```python
from build123d import *

# Parameters (mm, degrees)
BOSS_EXTRUDE2_START = -109.568605
BOSS_EXTRUDE2_DEPTH = 101.325087
CIRPATTERN1_COUNT   = 8


with BuildPart() as part:
    # Sketch3 → Revolve1 (revolve)
    with BuildSketch(Plane(origin=(0, 0, 0), x_dir=(0, 0, -1), z_dir=(1, 0, 0))):
        Polygon((0, 120), (0, 0), (10, 0), (10, 4.243518426), (8, 4.243518426), (8, 8.243518426), (10, 8.243518426), (10, 109.568605079), (8, 109.568605079), (8, 113.568605079), (10, 113.568605079), (10, 120), align=None)
    revolve(axis=Axis((0, 0, 0), (0, 1, 0)))

    # Sketch4 → Boss-Extrude2 (add)
    with BuildSketch(Plane.XZ.offset(BOSS_EXTRUDE2_START)):
        with BuildLine():
            Line((-1, 9.949874371), (-1, 10.949874371))
            Line((-1, 10.949874371), (1, 10.949874371))
            Line((1, 10.949874371), (1, 9.949874371))
            ThreePointArc((1, 9.949874371), (0, 10), (-1, 9.949874371))
        make_face()
    boss_extrude2 = extrude(amount=BOSS_EXTRUDE2_DEPTH)

    # CirPattern1: Boss-Extrude2 ×8 about axis
    cirpattern1_axis = Axis((0, 0, 0), (0, 1, 0))
    for i in range(1, CIRPATTERN1_COUNT):
        add(boss_extrude2.rotate(cirpattern1_axis, i * 360 / CIRPATTERN1_COUNT))


solid = part.part
```
Could you check a few things on this model? Use its own coordinates, in mm. A direction names the side the tool comes from. Round coordinates to 2 decimals unless told otherwise and drop trailing zeros. Loops run counter-clockwise (first coordinate to the right, second up) from the corner with the lowest first, then second, coordinate; pieces in that order, holes last. Notation, with made-up numbers: (55, 28.5) - (80, 28.5) arc R19 cw to (80, 36.5) - close; hole circle Ø4 at (-11.75, 81.25). An arc over 180 degrees is marked (long way). Answer as CSV lines item,"result".
1. I want a section at A-A on z = 0. List the corners of the cut face in (x, y) for me.
Filled in:
outline,"(-10.95, 8.24) - (-8, 8.24) - (-8, 4.24) - (-10, 4.24) - (-10, 0) - (10, 0) - (10, 4.24) - (8, 4.24) - (8, 8.24) - (10.95, 8.24) - (10.95, 109.57) - (8, 109.57) - (8, 113.57) - (10, 113.57) - (10, 120) - (-10, 120) - (-10, 113.57) - (-8, 113.57) - (-8, 109.57) - (-10.95, 109.57) - close"
2. Please list where these lines run through material, in increasing order: line 1 along Y through (x, z) = (1.25, -9); line 2 along X through (y, z) = (43, 8.25); line 3 along Z through (x, y) = (-8, 77.5). Write a range as [from, to].
Filled in:
line 1,"y = [0, 4.24], [8.24, 109.57], [113.57, 120]"
line 2,"x = [-7.24, -6.84], [-5.65, 5.65], [6.84, 7.24]"
line 3,"z = [-7.49, -6.59], [-6, 6], [6.59, 7.49]"
3. We'd pull the mould along Y, two halves only. Please class faces 6 (the face through (0, 0, 0)), 7 (the face through (3.789, 59.615, 9.254)), 8 (the face through (-8.2, 113.569, 0)): +Y half, -Y half, draft (parallel to the pull), parting line (faces both ways), or undercut.
Filled in:
face 6,"-Y half"
face 7,"draft"
face 8,"undercut"
4. On a 3-axis mill with a long thin cutter (end or side, diameter ignored), from which of +Z, -Z, +X, -X, +Y, -Y can I reach the whole of each face in a straight line? I mean faces 1 (the face through (-9.254, 59.615, 3.789)), 2 (the face through (9.76, 2.15, 2.17)), 3 (the face through (3.865, 59.615, -9.223)), 4 (the face through (-3.865, 59.615, 9.223)), 5 (the face through (7.81, 6.27, 1.73)). Say none if no direction works.
Filled in:
face 1,"-X, +Y, -Y"
face 2,"-Y"
face 3,"-Z, +Y, -Y"
face 4,"+Z, +Y, -Y"
face 5,"none"
5. For pin 1 Ø2 at (x, y) = (-6, 57.5) entering from -Z; pin 2 Ø0.5 at (x, y) = (-10.5, 78.5) entering from +Z; pin 3 Ø2 at (x, y) = (5.5, 104) entering from +Z, each with a flat end and sliding along its axis, tell me the tip position at first contact or that it passes through.
Filled in:
pin 1,"stops at z = -8.66"
pin 2,"stops at z = 1"
pin 3,"stops at z = 8.93"
6. I want a section at C-C on x = 0. List the corners of the cut face in (y, z) for me, then the cut area to 3 significant figures.
Filled in:
outline,"(0, -10) - (4.24, -10) - (4.24, -8) - (8.24, -8) - (8.24, -10.95) - (109.57, -10.95) - (109.57, -8) - (113.57, -8) - (113.57, -10) - (120, -10) - (120, 10) - (113.57, 10) - (113.57, 8) - (109.57, 8) - (109.57, 10.95) - (8.24, 10.95) - (8.24, 8) - (4.24, 8) - (4.24, 10) - (0, 10) - close"
area,"2,560 mm^2"
